from build123d import *

# Parameters (mm, degrees)
SKETCH1_W           = 17.805
SKETCH1_H           = 25
BOSS_EXTRUDE1_DEPTH = 3
FILLET1_R           = 2
BOSS_EXTRUDE3_DEPTH = 5
FILLET2_R           = 1
FILLET3_R           = 1
SKETCH3_R           = 1.5
CUT_EXTRUDE1_DEPTH  = 5
SKETCH7_W           = 15.61
SKETCH7_H           = 10
BOSS_EXTRUDE4_DEPTH = 30
BOSS_EXTRUDE5_DEPTH = 15.61
SKETCH9_R           = 1.5
CUT_EXTRUDE2_DEPTH  = 5


with BuildPart() as part:
    # Sketch1 → Boss-Extrude1 (new body)
    with BuildSketch(Plane(origin=(0, 0, 0), x_dir=(1, 0, 0), z_dir=(0, 1, 0))):
        Polygon((9.368218391, -4.75), (-8.436781609, -4.75), (-26.241781609, -4.75), (-38.436781609, -4.75), (-38.436781609, -9.75), (21.563218391, -9.75), (21.563218391, -4.75), align=None)
        with Locations((0.465718391, 7.75)):
            Rectangle(SKETCH1_W, SKETCH1_H)
        with Locations((-17.339281609, 7.75)):
            Rectangle(SKETCH1_W, SKETCH1_H)
    extrude(amount=BOSS_EXTRUDE1_DEPTH)

    # Fillet1
    fillet1_edges = [part.edges().sort_by_distance(p)[0] for p in [
        (-8.436781609, 0, 9.75),
    ]]
    fillet(fillet1_edges, radius=FILLET1_R)

    # Sketch2 → Boss-Extrude3 (add)
    with BuildSketch(Plane(origin=(21.563218391, 0, 0), x_dir=(0, 0, -1), z_dir=(1, 0, 0))):
        with BuildLine():
            Line((-29.75, 46.301270189), (-32.25, 41.97114317))
            ThreePointArc((-32.25, 41.97114317), (-15.77885683, 25.5), (-9.75, 3))
            Line((-9.75, 3), (-4.75, 3))
            ThreePointArc((-4.75, 3), (-11.448729811, 28), (-29.75, 46.301270189))
        make_face()
    boss_extrude3 = extrude(amount=-BOSS_EXTRUDE3_DEPTH)

    # Fillet2
    fillet2_edges = [part.edges().sort_by_distance(p)[0] for p in [
        (21.563218391, 0, 6.25),
        (21.563218391, 2.5, 9.75),
        (21.563218391, 1.5, 4.75),
        (21.563218391, 0.585786438, 9.164213562),
        (16.563218391, 25.5, 15.77885683),
        (19.063218391, 41.97114317, 32.25),
        (16.563218391, 28, 11.448729811),
        (19.063218391, 46.301270189, 29.75),
        (21.563218391, 25.5, 15.77885683),
        (21.563218391, 28, 11.448729811),
        (21.563218391, 44.13620668, 31),
    ]]
    fillet(fillet2_edges, radius=FILLET2_R)

    # Mirror3: Boss-Extrude3 across plane
    add(boss_extrude3.mirror(Plane(origin=(-8.436781609, 0, 0), x_dir=(0, 0, 1), z_dir=(1, 0, 0))))

    # Fillet3
    fillet3_edges = [part.edges().sort_by_distance(p)[0] for p in [
        (-38.436781609, 0, 6.25),
        (-38.436781609, 2.5, 9.75),
        (-38.436781609, 1.5, 4.75),
        (-38.436781609, 0.585786438, 9.164213562),
        (-38.436781609, 25.5, 15.77885683),
        (-35.936781609, 41.97114317, 32.25),
        (-38.436781609, 28, 11.448729811),
        (-38.436781609, 44.13620668, 31),
        (-35.936781609, 46.301270189, 29.75),
        (-33.436781609, 25.5, 15.77885683),
        (-33.436781609, 28, 11.448729811),
    ]]
    fillet(fillet3_edges, radius=FILLET3_R)

    # Sketch3 → Cut-Extrude1 (cut)
    with BuildSketch(Plane.XZ):
        with Locations(Location((-20.484687418, -8.75, 0), (0, 0, 270))):
            Circle(SKETCH3_R)
        with Locations(Location((-8.434877213, -16.25, 0), (0, 0, 270))):
            Circle(SKETCH3_R)
        with Locations(Location((3.614932992, -8.75, 0), (0, 0, 270))):
            Circle(SKETCH3_R)
    extrude(amount=-CUT_EXTRUDE1_DEPTH, mode=Mode.SUBTRACT)

    # Sketch7 → Boss-Extrude4 (add)
    with BuildSketch(Plane(origin=(0, 3, 0), x_dir=(1, 0, 0), z_dir=(0, 1, 0))):
        with Locations((-8.436781609, 0.25)):
            Rectangle(SKETCH7_W, SKETCH7_H)
    extrude(amount=BOSS_EXTRUDE4_DEPTH)

    # Sketch8 → Boss-Extrude5 (add)
    with BuildSketch(Plane.ZY.offset(16.241781609)):
        Polygon((-5.25, 33), (4.75, 43), (4.75, 33), align=None)
    extrude(amount=-BOSS_EXTRUDE5_DEPTH)

    # Sketch9 → Cut-Extrude2 (cut)
    with BuildSketch(Plane(origin=(0, 19.125, -19.125), x_dir=(1, 0, 0), z_dir=(0, 0.7071067811865461, -0.7071067811865489))):
        with Locations(Location((-11.436781609, -26.69328099, 0), (0, 0, 270))):
            Circle(SKETCH9_R)
        with Locations(Location((-5.436781609, -26.69328099, 0), (0, 0, 270))):
            Circle(SKETCH9_R)
    extrude(amount=-CUT_EXTRUDE2_DEPTH, mode=Mode.SUBTRACT)


solid = part.part
Can you work these out from the model? Positions are in its coordinate system, mm. A direction names the side the tool comes from. Coordinates: 2 decimals unless noted, no trailing zeros. Write each loop counter-clockwise with the first axis right and the second up, starting at its lowest first coordinate (ties: lowest second). Pieces come first, ordered by that corner, then holes. Notation, with made-up numbers: M 39.25,20.25 L 75.25,20.25 A22 cw 75.25,26.25 Z; hole C 84.5,-37 d10. An arc over 180 degrees is marked long. Use one line per item in the form item = value.
Q1. We'd pull the mould along X, two halves only. Please class faces 1 (the flat face through (-33.437, 26, 14)), 2 (the flat face through (-0.632, 19, 0)), 3 (the flat face through (18.59, 44.15, 30.99)), 4 (the flat face through (16.563, 26, 14)): +X half, -X half, draft (parallel to the pull), parting line (faces both ways), or undercut.
Model answer:
face_1 = undercut
face_2 = +X half
face_3 = draft
face_4 = undercut
Q2. I need wall thicknesses on line 1 along X through (y, z) = (1, -8.75); line 2 along Z through (x, y) = (-10.5, 15); line 3 along X through (y, z) = (22, -4). Which ranges of each line are inside material? Lowest first, please. Write a range as from..to.
Model answer:
line_1 = -26.24..-21.98, -18.98..2.11, 5.11..9.37
line_2 = -5.25..4.75
line_3 = -16.24..-0.63
Q3. If we section it at D-D (y = 36.5): State how many separate pieces and enclosed holes the cut face has, then the cut area to 3 significant figures.
Model answer:
separate_pieces = 3
enclosed_holes = 2
area = 150 mm^2
Q4. If we section it at C-C (x = -18): Write out the boundary of the cut face in (y, z).
Model answer:
outline = M 0,-20.25 L 3,-20.25 L 3,9.75 L 2,9.75 A2 ccw 0,7.75 Z
Q5. For P1, Ø24, axis at x = -1, z = -10, coming from the +Y side; P2, Ø12, axis at x = 14.5, y = 19, coming from the -Z side; P3, Ø0.9, axis at y = 1.5, z = -11.5, coming from the -X side, each with a flat end and sliding along its axis, tell me the tip position at first contact or that it passes through.
Model answer:
P1 = 40.25
P2 = 5.93
P3 = -26.24
Q6. If we section it at A-A (z = -16.25): Write out the boundary of the cut face in (x, y).
Model answer:
outline = M -26.24,0 L -9.93,0 L -9.93,3 L -26.24,3 Z; M -6.93,0 L 9.37,0 L 9.37,3 L -6.93,3 Z
Q7. For faces 5 (the flat face through (-9, 18, -5.25)), 6 (the flat face through (-26.242, 1, -8)), 7 (the flat face through (15, 1, 4.75)), which set-ups out of +Z, -Z, +X, -X, +Y, -Y let a thin tool reach every point of the face, with its end or its side?
Model answer:
face_5 = -Z, +X, -X, +Y
face_6 = -Z, -X, +Y, -Y
face_7 = -Z, +X, +Y, -Y
Q8. If we section it at B-B (z = -8.75): Write out the boundary of the cut face in (x, y), then the cut area to 3 significant figures.
Model answer:
outline = M -26.24,0 L -21.98,0 L -21.98,3 L -26.24,3 Z; M -18.98,0 L 2.11,0 L 2.11,3 L -18.98,3 Z; M 5.11,0 L 9.37,0 L 9.37,3 L 5.11,3 Z
area = 88.8 mm^2
